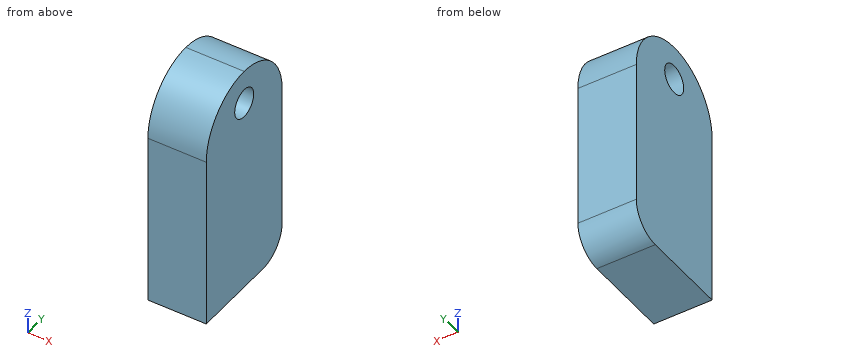
from build123d import *

# Parameters (mm, degrees)
F0_W     = 12.7
F0_H     = 50.8
F1_DEPTH = 25.4
F2_R     = 3.175
F3_DEPTH = 25.4
F4_R     = 12.7
F5_R     = 12.69999
F6_R     = 6.35


# Not quite as in the source:
# - a fillet or chamfer is up to 0.001 mm smaller than in the source, because OpenCascade refuses the exact size


with BuildPart() as f1:
    # F0 (on Front) → F1 (new body)
    with BuildSketch(Plane.XZ):
        Rectangle(F0_W, F0_H)
    extrude(amount=F1_DEPTH)

    # F2 (on face) → F3 (cut)
    with BuildSketch(Plane.YZ.offset(6.35)):
        with Locations((-12.7, 17.9132968187)):
            Circle(F2_R)
    extrude(amount=-F3_DEPTH, mode=Mode.SUBTRACT)

    # F4
    f4_edges = [f1.edges().sort_by_distance(p)[0] for p in [
        (0, -25.4, 25.4),
    ]]
    fillet(f4_edges, radius=F4_R)

    # F5 (radius 12.7 in the source; OpenCascade refuses exactly that, so slightly less here)
    f5_edges = [f1.edges().sort_by_distance(p)[0] for p in [
        (0, 0, 25.4),
    ]]
    fillet(f5_edges, radius=F5_R)

    # F6
    f6_edges = [f1.edges().sort_by_distance(p)[0] for p in [
        (0, 0, -25.4),
    ]]
    fillet(f6_edges, radius=F6_R)


solid = f1.part
Check sheet for the modelled part. Datum: model origin and axes. Units: mm. Give positions to 0.01 mm unless a question says otherwise; leave off trailing zeros. Loops run counter-clockwise (first coordinate to the right, second up) from the corner with the lowest first, then second, coordinate; pieces in that order, holes last. Notation, with made-up numbers: M -31,34 L -7,34 A22 ccw -7,44 Z; hole C 26,50 d5. An arc over 180 degrees is marked long. Answer as a JSON object with one key per item and string values. Group by question number.
Q1. Cross-section at D-D on y = -1.5. Record the cut outline in (x, z), then the cut area to 3 significant figures.
Q2. Cross-section at A-A on y = -13.25. Record the cut outline in (x, z), then the cut area to 3 significant figures.
Q3. Cross-section at B-B on z = 19. Record the cut outline in (x, y).
Q4. Material ranges on line 1 along Z through (x, y) = (-3.25, -12.7); line 2 along Z through (x, y) = (-4.25, -12); line 3 along Y through (x, z) = (4.5, 20.5), recorded low to high. Write a range as [from, to].
Q5. Go/stop test with a flat-tipped pin: P1, Ø5, axis at x = -3.5, y = -18.5, coming from the +Z side. Record where the tip stops, or that it passes through.
Evaluation:
{
 "1": {"outline": "M -6.35,-23.15 L 6.35,-23.15 L 6.35,18.69 L -6.35,18.69 Z", "area": "531 mm2"},
 "2": {"outline": "M -6.35,-25.4 L 6.35,-25.4 L 6.35,14.79 L -6.35,14.79 Z; M -6.35,21.04 L 6.35,21.04 L 6.35,25.39 L -6.35,25.39 Z", "area": "566 mm2"},
 "3": {"outline": "M -6.35,-23.73 L 6.35,-23.73 L 6.35,-15.68 L -6.35,-15.68 Z; M -6.35,-9.72 L 6.35,-9.72 L 6.35,-1.67 L -6.35,-1.67 Z"},
 "4": {"line 1": "z = [-25.4, 14.74], [21.09, 25.4]", "line 2": "z = [-25.4, 14.82], [21.01, 25.38]", "line 3": "y = [-22.72, -14.54], [-10.86, -2.68]"},
 "5": {"P1": "stops at z = 24.96"}
}
